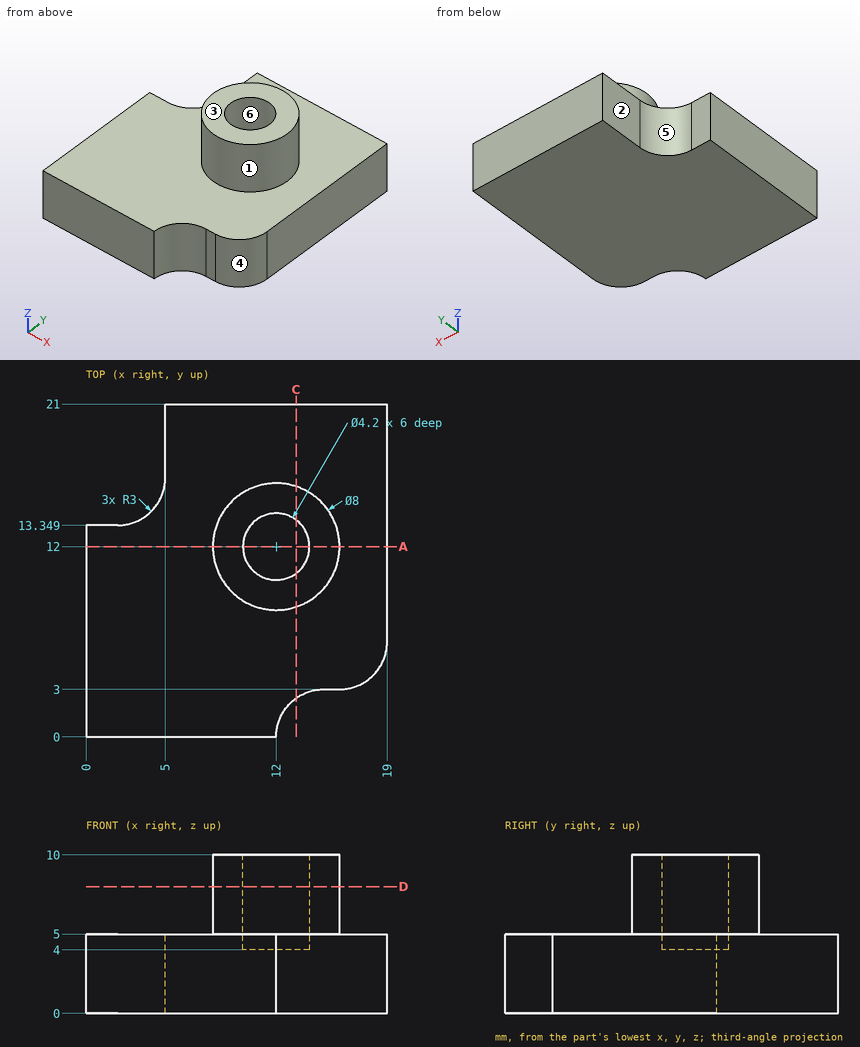
Answer from the drawing. Dimensions are ordinates in mm from the lowest x, y and z of the part. A direction names the side the tool comes from. Coordinates: 2 decimals unless noted, no trailing zeros. Order: outer loops, then holes, each group sorted by start corner. A loop starts at its lowest first (then second) coordinate and runs counter-clockwise, first axis right, second up. Notation, with made-up numbers: (-4.75, 64) - (45.25, 64) arc R25 ccw to (45.25, 99) - close; hole circle Ø11 at (76, 54.5). An arc over 180 degrees is marked (long way). Answer as a JSON object with one key per item and string values. Group by question number.
Item 1: Section A-A (y = 12) is taken. Give the vertices of the cut face in (x, z).
Item 2: Section C-C (x = 13.25) is taken. Give the vertices of the cut face in (y, z), plus the area to 3 significant figures.
Item 3: Flat-ended cylindrical pins translate along their axes: P1, Ø5, axis at y = 18.5, z = 2.5, coming from the -X side; P2, Ø2, axis at x = 3, y = 18, coming from the -Z side; P3, Ø0.5, axis at x = 15.5, z = 1.5, coming from the -Y side; P4, Ø1.6, axis at x = 1.5, z = 2, coming from the +Y side. Find the tip coordinate at first contact, or state that the pin passes through.
Item 4: The mould has two halves that part along Y. Classify the marked faces 4, 5 and 6: +Y half, -Y half, draft (parallel to the pull), parting line (faces both ways), or undercut.
Item 5: Section D-D (z = 8) is taken. Give the vertices of the cut face in (x, y), plus the area to 3 significant figures.
Item 6: Consider probe 1 along Y at (x, z) = (12, 7.3); probe 2 along Z at (x, y) = (13.25, 6.25); probe 3 along Y at (x, z) = (2, 3.5). Determine where each line is inside the solid, lowest interval first. Write a range as from..to.
Item 7: A tool of negligible diameter and unlimited length cuts with its end or side. For the marked faces 1, 2 and 3, from which of +Z, -Z, +X, -X, +Y, -Y can it reach the whole face along a straight path? Write none if from no direction.
Results are:
{
 "1": {"outline": "(0, 0) - (19, 0) - (19, 5) - (16, 5) - (16, 10) - (14.1, 10) - (14.1, 4) - (9.9, 4) - (9.9, 10) - (8, 10) - (8, 5) - (0, 5) - close"},
 "2": {"outline": "(2.44, 0) - (21, 0) - (21, 5) - (15.8, 5) - (15.8, 10) - (13.69, 10) - (13.69, 4) - (10.31, 4) - (10.31, 10) - (8.2, 10) - (8.2, 5) - (2.44, 5) - close", "area": "111 mm^2"},
 "3": {"P1": "stops at x = 4.98", "P2": "passes through", "P3": "stops at y = 3", "P4": "stops at y = 13.36"},
 "4": {"face 4": "-Y half", "face 5": "+Y half", "face 6": "undercut"},
 "5": {"outline": "circle Ø8 at (12, 12); hole circle Ø4.2 at (12, 12)", "area": "36.4 mm^2"},
 "6": {"probe 1": "y = 8..9.9, 14.1..16", "probe 2": "z = 0..5", "probe 3": "y = 0..13.35"},
 "7": {"face 1": "+Z", "face 2": "+Z, -Z, -X, +Y", "face 3": "+Z, +X, -X, +Y, -Y"}
}
